from build123d import *

# Parameters (mm, degrees)
F0_W      = 1016
F0_H      = 508
F1_DEPTH  = 101.6
F4_W      = 237.9516797066
F4_H      = 381
F4_W_2    = 270.0483202934
F5_DEPTH  = 76.2
F5_FACE_W = 508
F5_FACE_H = 381
F6_DEPTH  = 149.86
F6_TAPER  = 45
F7_R      = 63.5
F8_DEPTH  = 76.2


# Not quite as in the source:
# - the program builds the solid bodies; features that only make, move or delete a surface that nothing else refers to are left out


with BuildPart() as f1:
    # F0 (on Top) → F1 (new body)
    with BuildSketch(Plane.XY):
        Rectangle(F0_W, F0_H)
    extrude(amount=F1_DEPTH)

    # F4 (on face) → F5 (join)
    with BuildSketch(Plane.XY.offset(101.6)):
        with Locations((118.9758398533, -63.5)):
            Rectangle(F4_W, F4_H)
        with Locations((-135.0241601467, -63.5)):
            Rectangle(F4_W_2, F4_H)
    extrude(amount=F5_DEPTH)

    # F5_face (on face) → F6 (join, symmetric)
    with BuildSketch(Plane(origin=(-16.0483202934, -63.5, 177.8), x_dir=(1, 0, 0), z_dir=(0, 0, 1))):
        Rectangle(F5_FACE_W, F5_FACE_H)
    extrude(amount=F6_DEPTH, both=True, taper=F6_TAPER)

    # F7 (on face) → F8 (cut)
    with BuildSketch(Plane(origin=(0, 152.4, 152.4), x_dir=(-1, 0, 0), z_dir=(0, 0.7071067812, 0.7071067812))):
        with Locations((10.2272699534, 145.9400733915)):
            Circle(F7_R)
    extrude(amount=-F8_DEPTH, mode=Mode.SUBTRACT)


solid = f1.part
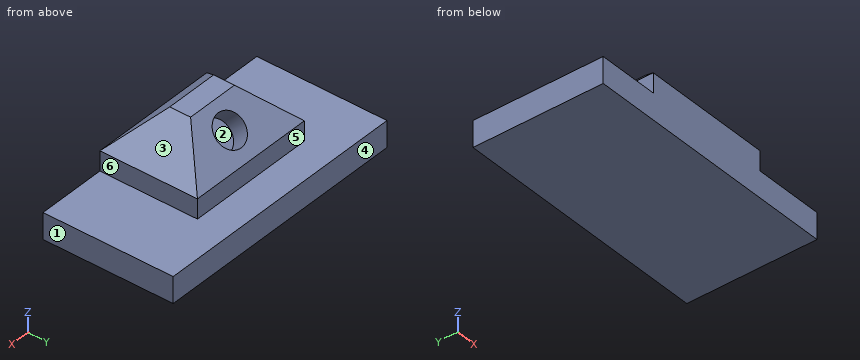
Could you check a few things on this model? Use its own coordinates, in mm. Face numbers are marked on the shaded views. A direction names the side the tool comes from. Coordinates: 2 decimals unless noted, no trailing zeros. Loops run counter-clockwise (first coordinate to the right, second up) from the corner with the lowest first, then second, coordinate; pieces in that order, holes last.
1. I need wall thicknesses on L1, parallel to Z at x = -390, y = -42; L2, parallel to Y at x = -195, z = 150.5; L3, parallel to X at y = 122.5, z = 176. Which ranges of each line are inside material? Lowest first, please.
2. Imagine slicing it at B-B (x = 110). Please give me the cut outline in (y, z), and give its area (3 significant figures).
3. For the marked faces 4, 5 and 6, which set-ups out of +Z, -Z, +X, -X, +Y, -Y let a thin tool reach every point of the face, with its end or its side?
4. We'd pull the mould along Z, two halves only. Please class the marked faces 1, 2 and 3: released by +Z, released by -Z, zero draft, split by the parting line, or undercut.
5. Imagine slicing it at C-C (y = -189). Please give me the cut outline in (x, z).
6. Imagine slicing it at A-A (y = -87.5). Please give me the cut outline in (x, z).
7. For P1, Ø23, axis at y = -120.5, z = 152.5, coming from the -X side; P2, Ø23, axis at x = -76.5, z = 151.5, coming from the +Y side; P3, Ø12, axis at x = 0, z = 273, coming from the +Y side, each with a flat end and sliding along its axis, tell me the tip position at first contact or that it passes through.
8. Imagine slicing it at D-D (x = 291.5). Please give me the cut outline in (y, z).
Computed values:
1. L1: z = 0 to 101.6
1. L2: y = -254 to 127
1. L3: x = -270.05 to 237.95
2. outline: (-254, 0) - (254, 0) - (254, 101.6) - (127, 101.6) - (127, 177.8) - (-0.95, 305.75) - (-126.05, 305.75) - (-254, 177.8) - close
2. area: 113,000 mm2
3. face 4: +Z, -Z, +X, -X, +Y
3. face 5: +Z, +X, -X, +Y
3. face 6: +Z, +X, +Y, -Y
4. face 1: zero draft
4. face 2: undercut
4. face 3: released by +Z
5. outline: (-508, 0) - (508, 0) - (508, 101.6) - (237.95, 101.6) - (237.95, 177.8) - (172.95, 242.8) - (-205.05, 242.8) - (-270.05, 177.8) - (-270.05, 101.6) - (-508, 101.6) - close
6. outline: (-508, 0) - (508, 0) - (508, 101.6) - (237.95, 101.6) - (237.95, 177.8) - (88.09, 327.66) - (-120.19, 327.66) - (-270.05, 177.8) - (-270.05, 101.6) - (-508, 101.6) - close
7. P1: stops at x = -270.05
7. P2: stops at y = 127
7. P3: stops at y = -15.84
8. outline: (-254, 0) - (254, 0) - (254, 101.6) - (-254, 101.6) - close
